```python
from build123d import *

# Parameters (mm, degrees)
F3_DEPTH = 10.570714
F4_R     = 10


with BuildPart() as f1:
    # F0 (on Front) → F1 (revolve)
    with BuildSketch(Plane.XZ):
        with BuildLine():
            Line((0, 10.570714), (0, 14))
            ThreePointArc((0, 14), (-6.297257, 10.056887), (-5.5, 2.669873))
            Line((-5.5, 2.669873), (-5.5, 0))
            Line((-5.5, 0), (-3.5, 0))
            Line((-3.5, 0), (-3.5, 10.570714))
            Line((-3.5, 10.570714), (0, 10.570714))
        make_face()
    revolve(axis=Axis((0, 0, 5.285357), (0, 0, 1)))

    # F2 (on face) → F3 (cut, through all)
    with BuildSketch(Plane(origin=(0, 0, 0), x_dir=(1, 0, 0), z_dir=(0, 0, -1))):
        with BuildLine():
            Line((-2.020726, -3.5), (0, -3.5))
            ThreePointArc((0, -3.5), (-1.75, -3.031089), (-3.031089, -1.75))
            Line((-3.031089, -1.75), (-2.020726, -3.5))
        make_face()
        with BuildLine():
            Line((-4.041452, 0), (-3.031089, -1.75))
            ThreePointArc((-3.031089, -1.75), (-3.5, 0), (-3.031089, 1.75))
            Line((-3.031089, 1.75), (-4.041452, 0))
        make_face()
        with BuildLine():
            Line((-2.020726, 3.5), (-3.031089, 1.75))
            ThreePointArc((-3.031089, 1.75), (-1.75, 3.031089), (0, 3.5))
            Line((0, 3.5), (-2.020726, 3.5))
        make_face()
        with BuildLine():
            ThreePointArc((0, 3.5), (1.75, 3.031089), (3.031089, 1.75))
            Line((3.031089, 1.75), (2.020726, 3.5))
            Line((2.020726, 3.5), (0, 3.5))
        make_face()
        with BuildLine():
            ThreePointArc((3.5, 0), (3.38074, -0.905867), (3.031089, -1.75))
            Line((3.031089, -1.75), (4.041452, 0))
            Line((4.041452, 0), (3.031089, 1.75))
            ThreePointArc((3.031089, 1.75), (3.38074, 0.905867), (3.5, 0))
        make_face()
        with BuildLine():
            Line((0, -3.5), (2.020726, -3.5))
            Line((2.020726, -3.5), (3.031089, -1.75))
            ThreePointArc((3.031089, -1.75), (1.75, -3.031089), (0, -3.5))
        make_face()
    extrude(amount=-F3_DEPTH, mode=Mode.SUBTRACT)

    # F4
    f4_edges = [f1.edges().sort_by_distance(p)[0] for p in [
        (5.5, 0, 2.669873),
    ]]
    fillet(f4_edges, radius=F4_R)


solid = f1.part
```
Design review of the part built by this model. Coordinates are the model's own, in mm. Coordinates: 2 decimals unless noted, no trailing zeros.
1) To check wall thickness, follow L1, parallel to Y at x = 3.75, z = 7; L2, parallel to Y at x = 2.5, z = 8; L3, parallel to X at y = -3.25, z = 3. State the ranges of each line that lie inside material, in increasing order.
2) Mouldability with a two-part tool opening along Y and no side actions: class faces 1 (the flat face through (-3, -1.8, 5.2)), 2 (the flat face through (0, 4, 0)) as +Y half, -Y half, draft (parallel to the pull), parting line (faces both ways), or undercut.
3) Insertion check: pin 1 (6 mm diameter, centred on y = 3, z = 9, fed in from +X); pin 2 (4 mm diameter, centred on y = 4, z = 9, fed in from -X); pin 3 (6 mm diameter, centred on x = 1.5, z = 11, fed in from -Y). Each pin has a flat end and moves straight along its axis. Give the tip position at first contact, or say it passes through.
Check result:
1. L1: y = -5.91 to -0.5, 0.5 to 5.91
1. L2: y = -6.46 to -2.67, 2.67 to 6.46
1. L3: x = -4.99 to -2.17, 2.17 to 4.99
2. face 1: undercut
2. face 2: draft
3. pin 1: stops at x = 6.97
3. pin 2: stops at x = -6.55
3. pin 3: stops at y = -6.88
